Read the model definition and answer for the solid it produces. Units are mm, in the model's axes. Round coordinates to 2 decimals unless told otherwise and drop trailing zeros. Write each loop counter-clockwise with the first axis right and the second up, starting at its lowest first coordinate (ties: lowest second). Pieces come first, ordered by that corner, then holes. Notation, with made-up numbers: (28, -32) - (32, -32) arc R17 cw to (32, -13) - close; hole circle Ø3 at (7, 40.25). An arc over 180 degrees is marked (long way). Answer as CSV lines item,"result". Start each with the question number.
1) Each of these flat-tipped pins is pushed along its axis until it touches: pin 1 (12.5 mm diameter, centred on x = 38.1, z = -11.176, fed in from -Y); pin 2 (4 mm diameter, centred on x = -147, y = 8, fed in from -Z); pin 3 (6.5 mm diameter, centred on y = 9.5, z = -44.5, fed in from +X); pin 4 (1 mm diameter, centred on y = 7.5, z = 70, fed in from -X). Where does it stop, or does it pass through?
2) Find section A-A on x = -110. Determine the outline of the cut face in (y, z).
3) Consider line 1 along Z through (x, y) = (-106, 6.75); line 2 along Z through (x, y) = (-125, 5); line 3 along X through (y, z) = (2.25, 112.5). Determine where each line is inside the solid, lowest interval first.
4) Find section C-C on z = 4. Determine the outline of the cut face in (x, y), then the cut area to 3 significant figures.
5) Find section B-B on x = -46.5. Determine the outline of the cut face in (y, z).
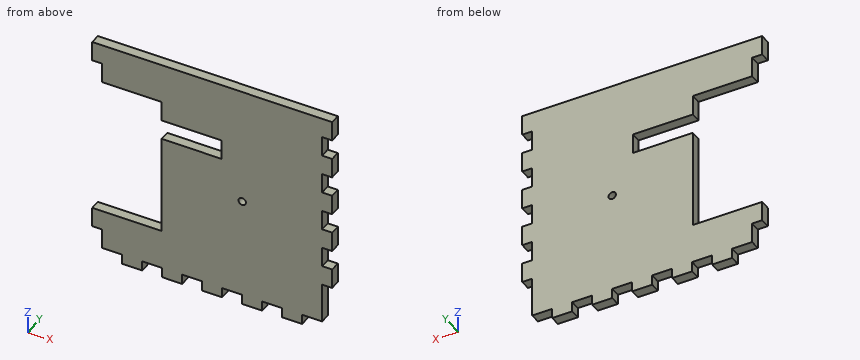
from build123d import *

# Parameters (mm, degrees)
SKETCH1_W               = 279.4
SKETCH1_H               = 279.4
BOSS_EXTRUDE1_DEPTH     = 12.7
SKETCH2_W               = 25.4
SKETCH2_H               = 12.7
BOSS_EXTRUDE2_DEPTH     = 12.7
LPATTERN1_COUNT         = 5
LPATTERN1_PITCH         = 50.8
MIRROR1_COPY_1_SKETCH_W = 25.4
MIRROR1_COPY_1_SKETCH_H = 12.7
MIRROR1_COPY_1_DEPTH    = 12.7
MIRROR1_COPY_2_SKETCH_W = 25.4
MIRROR1_COPY_2_SKETCH_H = 12.7
MIRROR1_COPY_2_DEPTH    = 12.7
MIRROR1_COPY_3_SKETCH_W = 25.4
MIRROR1_COPY_3_SKETCH_H = 12.7
MIRROR1_COPY_3_DEPTH    = 12.7
MIRROR1_COPY_4_SKETCH_W = 25.4
MIRROR1_COPY_4_SKETCH_H = 12.7
MIRROR1_COPY_4_DEPTH    = 12.7
SKETCH3_W               = 25.4
SKETCH3_H               = 12.7
BOSS_EXTRUDE3_DEPTH     = 12.7
LPATTERN2_COUNT         = 5
LPATTERN2_PITCH         = 50.8
SKETCH6_R               = 4.7625
CUT_EXTRUDE1_DEPTH      = 13.7
SKETCH8_W               = 88.066093183
SKETCH8_H               = 177.8
CUT_EXTRUDE3_DEPTH      = 13.7
SKETCH9_W               = 25.4
SKETCH9_H               = 12.7
BOSS_EXTRUDE4_DEPTH     = 12.7
SKETCH11_W              = 25.4
SKETCH11_H              = 12.7
CUT_EXTRUDE4_DEPTH      = 76.2


with BuildPart() as part:
    # Sketch1 → Boss-Extrude1 (new body)
    with BuildSketch(Plane(origin=(0, 0, 0), x_dir=(1, 0, 0), z_dir=(0, 1, 0))):
        Rectangle(SKETCH1_W, SKETCH1_H)
    extrude(amount=BOSS_EXTRUDE1_DEPTH)

    # Sketch2 → Boss-Extrude2 (add)
    with BuildSketch(Plane(origin=(139.7, 0, 0), x_dir=(0, 0, -1), z_dir=(1, 0, 0))):
        with Locations((-127, 6.35)):
            Rectangle(SKETCH2_W, SKETCH2_H)
    boss_extrude2 = extrude(amount=BOSS_EXTRUDE2_DEPTH)

    # LPattern1: Boss-Extrude2 ×5
    with Locations(*[(0, 0, -i * LPATTERN1_PITCH) for i in range(1, LPATTERN1_COUNT)]):
        add(boss_extrude2)

    # Mirror1: Boss-Extrude2 across plane
    add(boss_extrude2.mirror(Plane(origin=(0, 0, 0), x_dir=(0, 0, 1), z_dir=(1, 0, 0))))

    # Mirror1 copy 1 sketch → Mirror1 copy 1 (add)
    with BuildSketch(Plane(origin=(-139.7, 0, -50.8), x_dir=(0, 0, -1), z_dir=(-1, 0, 0))):
        with Locations((-127, -6.35)):
            Rectangle(MIRROR1_COPY_1_SKETCH_W, MIRROR1_COPY_1_SKETCH_H)
    extrude(amount=MIRROR1_COPY_1_DEPTH)

    # Mirror1 copy 2 sketch → Mirror1 copy 2 (add)
    with BuildSketch(Plane(origin=(-139.7, 0, -101.6), x_dir=(0, 0, -1), z_dir=(-1, 0, 0))):
        with Locations((-127, -6.35)):
            Rectangle(MIRROR1_COPY_2_SKETCH_W, MIRROR1_COPY_2_SKETCH_H)
    extrude(amount=MIRROR1_COPY_2_DEPTH)

    # Mirror1 copy 3 sketch → Mirror1 copy 3 (add)
    with BuildSketch(Plane(origin=(-139.7, 0, -152.4), x_dir=(0, 0, -1), z_dir=(-1, 0, 0))):
        with Locations((-127, -6.35)):
            Rectangle(MIRROR1_COPY_3_SKETCH_W, MIRROR1_COPY_3_SKETCH_H)
    extrude(amount=MIRROR1_COPY_3_DEPTH)

    # Mirror1 copy 4 sketch → Mirror1 copy 4 (add)
    with BuildSketch(Plane(origin=(-139.7, 0, -203.2), x_dir=(0, 0, -1), z_dir=(-1, 0, 0))):
        with Locations((-127, -6.35)):
            Rectangle(MIRROR1_COPY_4_SKETCH_W, MIRROR1_COPY_4_SKETCH_H)
    extrude(amount=MIRROR1_COPY_4_DEPTH)

    # Sketch3 → Boss-Extrude3 (add)
    with BuildSketch(Plane(origin=(0, 0, -139.7), x_dir=(-1, 0, 0), z_dir=(0, 0, -1))):
        with Locations((-101.6, 6.35)):
            Rectangle(SKETCH3_W, SKETCH3_H)
    boss_extrude3 = extrude(amount=BOSS_EXTRUDE3_DEPTH)

    # LPattern2: Boss-Extrude3 ×5
    with Locations(*[(-i * LPATTERN2_PITCH, 0, 0) for i in range(1, LPATTERN2_COUNT)]):
        add(boss_extrude3)

    # Sketch6 → Cut-Extrude1 (cut, through all)
    with BuildSketch(Plane(origin=(0, 12.7, 0), x_dir=(1, 0, 0), z_dir=(0, 1, 0))):
        with Locations((38.1, 11.176)):
            Circle(SKETCH6_R)
    extrude(amount=-CUT_EXTRUDE1_DEPTH, mode=Mode.SUBTRACT)

    # Sketch8 → Cut-Extrude3 (cut, through all)
    with BuildSketch(Plane(origin=(0, 12.7, 0), x_dir=(1, 0, 0), z_dir=(0, 1, 0))):
        with Locations((-108.366953408, 0)):
            Rectangle(SKETCH8_W, SKETCH8_H)
    extrude(amount=-CUT_EXTRUDE3_DEPTH, mode=Mode.SUBTRACT)

    # Sketch9 → Boss-Extrude4 (add)
    with BuildSketch(Plane.ZY.offset(139.7)):
        with Locations((-101.6, 6.35)):
            Rectangle(SKETCH9_W, SKETCH9_H)
    extrude(amount=BOSS_EXTRUDE4_DEPTH)

    # Sketch11 → Cut-Extrude4 (cut)
    with BuildSketch(Plane.ZY.offset(64.333906817)):
        with Locations((50.8, 6.35)):
            Rectangle(SKETCH11_W, SKETCH11_H)
    extrude(amount=-CUT_EXTRUDE4_DEPTH, mode=Mode.SUBTRACT)


solid = part.part
Check values:
1,pin 1,"stops at y = 0"
1,pin 2,"stops at z = -114.3"
1,pin 3,"stops at x = 139.7"
1,pin 4,"stops at x = -64.33"
2,outline,"(0, -152.4) - (12.7, -152.4) - (12.7, -88.9) - (0, -88.9) - close; (0, 88.9) - (12.7, 88.9) - (12.7, 139.7) - (0, 139.7) - close"
3,line 1,"z = -152.4 to -88.9, 88.9 to 139.7"
3,line 2,"z = -139.7 to -88.9, 88.9 to 139.7"
3,line 3,"x = -139.7 to 139.7"
4,outline,"(-64.33, 0) - (139.7, 0) - (139.7, 12.7) - (-64.33, 12.7) - close"
4,area,"2,590 mm^2"
5,outline,"(0, -152.4) - (12.7, -152.4) - (12.7, 38.1) - (0, 38.1) - close; (0, 63.5) - (12.7, 63.5) - (12.7, 139.7) - (0, 139.7) - close"
